The listing builds one solid part. Answer for the finished solid, in the listing's coordinates (mm). Face numbers are marked on the shaded views. A direction names the side the tool comes from. Give positions to 0.01 mm unless a question says otherwise; leave off trailing zeros. Order: outer loops, then holes, each group sorted by start corner. A loop starts at its lowest first (then second) coordinate and runs counter-clockwise, first axis right, second up. Notation, with made-up numbers: (60.25, 74.5) - (107.25, 74.5) arc R26 ccw to (107.25, 97.5) - close; hole circle Ø11 at (14.25, 47.25). An arc over 180 degrees is marked (long way). Use a Markdown table: item, result. Add a question column.
1) For the marked faces 1, 2, 3, 4 and 5, determine the directions among +Z, -Z, +X, -X, +Y, -Y from which every point of the face is accessible in a straight line to the end or side of a thin tool.
2) Find section A-A, the plane x = 25.5. Determine the outline of the cut face in (y, z).
3) The mould has two halves that part along Y. Classify the marked faces 6, 7 and 8: released by +Y, released by -Y, zero draft, split by the parting line, or undercut.
4) Flat-ended cylindrical pins translate along their axes: pin 1 (1.3 mm diameter, centred on y = 1, z = -1.5, fed in from -X); pin 2 (4 mm diameter, centred on x = 21.5, z = 4, fed in from -Y); pin 3 (1.5 mm diameter, centred on y = -3.5, z = 4, fed in from +X) (3 decimals). Find the tip coordinate at first contact, or state that the pin passes through.
5) Find section B-B, the plane x = 17. Determine the outline of the cut face in (y, z), plus the area to 3 significant figures.
6) Straight lines are drawn through the part: line 1 (X direction, y = 2.5, z = -3.75) (3 decimals); line 2 (X direction, y = -2, z = -3.5) (3 decimals); line 3 (X direction, y = 0, z = 5.25). For each, find the intervals that lie inside material, in ascending order.
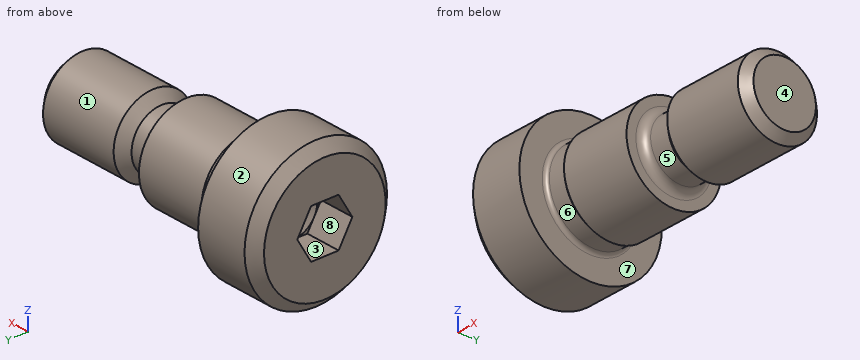
from build123d import *

# Parameters (mm, degrees)
HEX_2_DEPTH = 3.5814


# Read off the part's stored shape, not the designer's step: ThreadSchematic
with BuildPart() as part:
    # ThreadSchematic outline → ThreadSchematic (revolve)
    with BuildSketch(Plane.YX):
        with BuildLine():
            Line((0, 28.575), (0, 0))
            Line((0, 0), (6.096, 0))
            Line((6.096, 0), (7.1374, 1.0414))
            Line((7.1374, 1.0414), (7.1374, 6.35))
            Line((7.1374, 6.35), (4.8514, 6.35))
            ThreePointArc((4.8514, 6.35), (4.581992316, 6.461592316), (4.4704, 6.731))
            Line((4.4704, 6.731), (4.4704, 8.4455))
            Line((4.4704, 8.4455), (4.7371, 8.7122))
            Line((4.7371, 8.7122), (4.7371, 15.875))
            Line((4.7371, 15.875), (3.7973, 15.875))
            ThreePointArc((3.7973, 15.875), (3.24052412, 16.10562412), (3.0099, 16.6624))
            Line((3.0099, 16.6624), (3.0099, 18.6944))
            Line((3.0099, 18.6944), (3.96875, 19.65325))
            Line((3.96875, 19.65325), (3.96875, 27.73553))
            Line((3.96875, 27.73553), (3.12928, 28.575))
            Line((3.12928, 28.575), (0, 28.575))
        make_face()
    revolve(axis=Axis((0, 0, 0), (1, 0, 0)))

    # Sketch2 → PreBroach (revolve, cut)
    with BuildSketch(Plane.XY, mode=Mode.PRIVATE) as prebroach_sk:
        Polygon((0, 2.3876), (3.5814, 2.3876), (4.959881503, 0), (0, 0), align=None)
    revolve(prebroach_sk.sketch.rotate(Axis((0, 0, 0), (1, 0, 0)), 90), axis=Axis((0, 0, 0), (1, 0, 0)), mode=Mode.SUBTRACT)

    # Sketch3 → Hex 2 (cut)
    with BuildSketch(Plane.ZY):
        Polygon((-2.3876, -1.378481503), (-2.3876, 1.378481503), (0, 2.756963005), (2.3876, 1.378481503), (2.3876, -1.378481503), (0, -2.756963005), align=None)
    extrude(amount=-HEX_2_DEPTH, mode=Mode.SUBTRACT)


solid = part.part
The answers:
| question | item | result |
|---|---|---|
| 1 | face 1 | +X |
| 1 | face 2 | +X, -X |
| 1 | face 3 | -X |
| 1 | face 4 | +Z, -Z, +X, +Y, -Y |
| 1 | face 5 | none |
| 2 | outline | circle Ø7.94 at (0, 0) |
| 3 | face 6 | split by the parting line |
| 3 | face 7 | zero draft |
| 3 | face 8 | undercut |
| 4 | pin 1 | x = 3.58 |
| 4 | pin 2 | y = -3.43 |
| 4 | pin 3 | x = 15.875 |
| 5 | outline | circle Ø6.02 at (0, 0) |
| 5 | area | 28.5 mm2 |
| 6 | line 1 | 0 to 6.568, 8.482 to 15.875 |
| 6 | line 2 | 0 to 15.875 |
| 6 | line 3 | 0 to 6.35 |
